```python
from build123d import *

# Parameters (mm, degrees)
NUT_DEPTH       = 1.8
THREAD_SKETCH_W = 3.8
THREAD_SKETCH_H = 1.5


with BuildPart() as part:
    # Nut Sketch → Nut (new body)
    with BuildSketch(Plane(origin=(0, 0, 0), x_dir=(0, 0, -1), z_dir=(1, 0, 0))):
        Polygon((3.175426481, 0), (1.58771324, 2.75), (-1.58771324, 2.75), (-3.175426481, 0), (-1.58771324, -2.75), (1.58771324, -2.75), align=None)
    extrude(amount=NUT_DEPTH)

    # Thread Sketch → Thread (revolve, cut)
    with BuildSketch(Plane.XY, mode=Mode.PRIVATE) as thread_sk:
        with Locations((0.9, 0.75)):
            Rectangle(THREAD_SKETCH_W, THREAD_SKETCH_H)
    revolve(thread_sk.sketch.rotate(Axis((-1000, 0, 0), (1, 0, 0)), 270), axis=Axis((-1000, 0, 0), (1, 0, 0)), mode=Mode.SUBTRACT)


solid = part.part
```
Geometry: final body of the model. Coordinates: model frame, mm. Coordinates: 2 decimals unless noted, no trailing zeros. Order: outer loops, then holes, each group sorted by start corner. A loop starts at its lowest first (then second) coordinate and runs counter-clockwise, first axis right, second up. Notation, with made-up numbers: (-15, 22.5) -> (39, 22.5) arc R27 ccw to (39, 51.5) -> close; hole circle Ø2 at (-4.5, 80). An arc over 180 degrees is marked (long way). Answer in a Markdown table with one row per item.
Item 1: Ray query, L1, parallel to Y at x = 0.55, z = 0; L2, parallel to Y at x = 1.6, z = 0.5; L3, parallel to Z at x = 1.35, y = -0.25. Return the intervals inside material, ascending.
Return value:
| item | result |
|---|---|
| L1 | y = -2.75 to -1.5, 1.5 to 2.75 |
| L2 | y = -2.75 to -1.41, 1.41 to 2.75 |
| L3 | z = -3.03 to -1.48, 1.48 to 3.03 |
Item 2: Section B-B on x = 0.2. Output: boundary loops of the cut face in (y, z).
Return value:
| item | result |
|---|---|
| outline | (-2.75, -1.59) -> (0, -3.18) -> (2.75, -1.59) -> (2.75, 1.59) -> (0, 3.18) -> (-2.75, 1.59) -> close; hole circle Ø3 at (0, 0) |
Item 3: Section C-C on y = -0.2. Output: boundary loops of the cut face in (x, z).
Return value:
| item | result |
|---|---|
| outline | (0, -3.06) -> (1.8, -3.06) -> (1.8, -1.49) -> (0, -1.49) -> close; (0, 1.49) -> (1.8, 1.49) -> (1.8, 3.06) -> (0, 3.06) -> close |
Item 4: Section A-A on z = 0. Output: boundary loops of the cut face in (x, y).
Return value:
| item | result |
|---|---|
| outline | (0, -2.75) -> (1.8, -2.75) -> (1.8, -1.5) -> (0, -1.5) -> close; (0, 1.5) -> (1.8, 1.5) -> (1.8, 2.75) -> (0, 2.75) -> close |
Item 5: Section D-D on z = -2. Output: boundary loops of the cut face in (x, y).
Return value:
| item | result |
|---|---|
| outline | (0, -2.04) -> (1.8, -2.04) -> (1.8, 2.04) -> (0, 2.04) -> close |
Item 6: Draft query along Z for faces 1 (the flat face through (0, 1.3, -1.4)), 2 (the cylindrical face through (0.91, 0.45, -1.43)), 3 (the flat face through (0.887, 1.394, 2.37)), 4 (the flat face through (0.887, -1.394, -2.37)). Return one class per face: released by +Z, released by -Z, zero draft, split by the parting line, or undercut.
Return value:
| item | result |
|---|---|
| face 1 | zero draft |
| face 2 | undercut |
| face 3 | released by +Z |
| face 4 | released by -Z |
